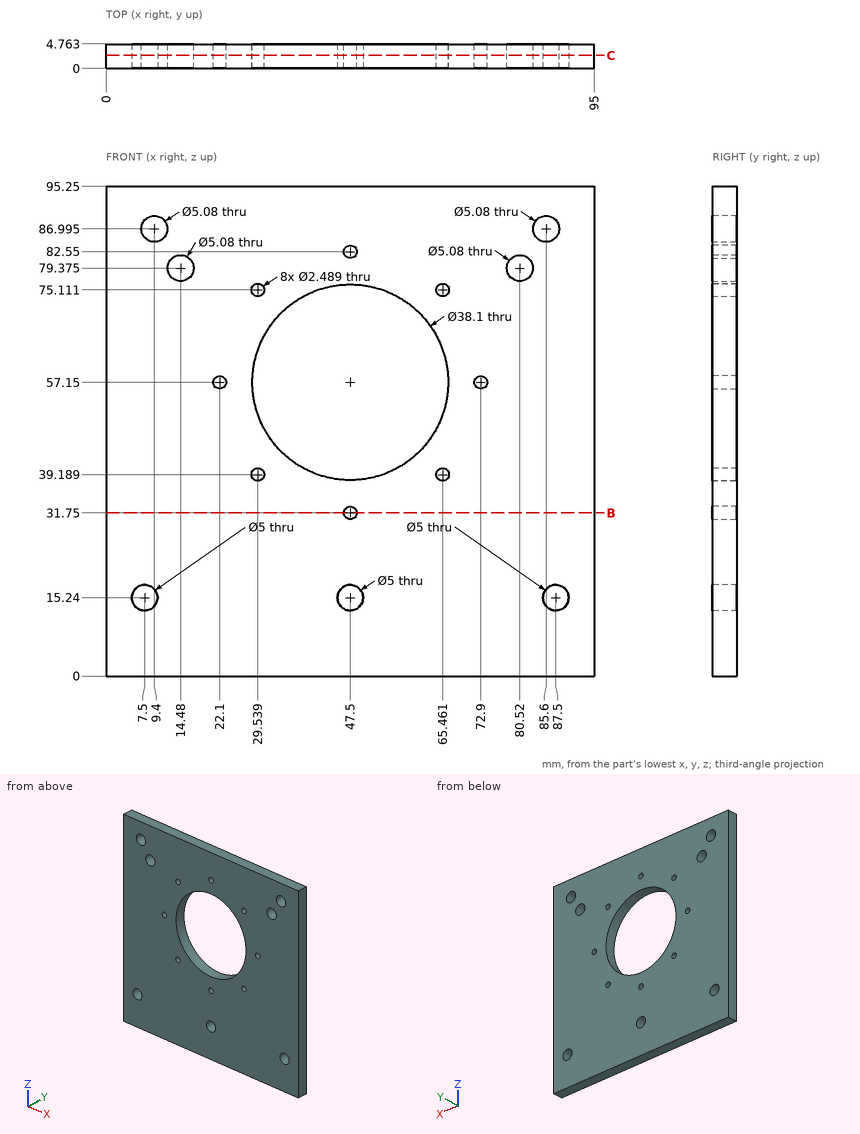
Geometry: see drawing. Coordinates: mm, zero at the bounding-box minimum. Round coordinates to 2 decimals unless told otherwise and drop trailing zeros. Order: outer loops, then holes, each group sorted by start corner. A loop starts at its lowest first (then second) coordinate and runs counter-clockwise, first axis right, second up. Notation, with made-up numbers: (-15, 10) -> (35, 10) arc R19 cw to (35, 23) -> close; hole circle Ø5 at (46, 13.25). An arc over 180 degrees is marked (long way). Write each question's results on one line, items separated by ' | '.
Q1. Ray query, line 1 along X through (y, z) = (4.1, 17) (1 decimal); line 2 along X through (y, z) = (3.85, 78.5) (1 decimal); line 3 along Z through (x, y) = (89, 0.75). Return the intervals inside material, ascending.
Response values:
line 1: 0 to 5.7, 9.3 to 45.7, 49.3 to 85.7, 89.3 to 95 | line 2: 0 to 12.1, 16.9 to 78.1, 82.9 to 95 | line 3: 0 to 13.24, 17.24 to 95.25
Q2. Section query C-C (y = 2.55). Count the separate pieces of the cut face and the enclosed holes in it, and give its area (3 significant figures).
Response values:
separate pieces: 1 | enclosed holes: 16 | area: 7,730 mm²
Q3. Section query B-B (z = 31.75). Output: boundary loops of the cut face in (x, y) (1 decimal).
Response values:
outline: (0, 0) -> (46.3, 0) -> (46.3, 4.8) -> (0, 4.8) -> close; (48.7, 0) -> (95, 0) -> (95, 4.8) -> (48.7, 4.8) -> close
Q4. Pin query (flat end, axial travel): pin 1 Ø3 at (x, z) = (47.5, 82.55) entering from -Y. Return the tip coordinate at first contact, or that it passes through.
Response values:
pin 1: y = 0
